Autodesk Inventor part; units mm, degrees
ref_plane "Work Plane1" through (0, 0, 0) normal (0.7071, 0.7071, 0) x (0, 0, 1)
ref_plane "XZ Plane" through (0, 0, 0) normal (0, 1, 0) x (-1, 0, 0)
ref_plane "XY Plane" through (0, 0, 0) normal (0, 0, 1) x (1, 0, 0)
sketch "Sketch1" plane through (0, 0, 0) normal (0, 0, 1) x (1, 0, 0)
  circle A0 centre (0, 0) radius 17.5
  dimension "d0" = 35
extrude "Extrusion1" add sketch "Sketch1" along normal blind 4
sketch "Sketch2" plane through (0, 0, 4) normal (0, 0, 1) x (1, 0, 0)
  circle A0 centre (0, 0) radius 7.625
  dimension "d3" = 15.25
extrude "Extrusion2" add sketch "Sketch2" along normal blind 5
chamfer "Chamfer1" distance 0.5 angle 45 1 edges at (-7.625, 0, 9)
sketch "Sketch3" plane through (0, 0, 0) normal (0, 0, -1) x (-1, 0, 0)
  line L0 (-7.4, -7.4) -> (7.4, -7.4)
  line L1 (7.4, -7.4) -> (7.4, 7.4)
  line L2 (7.4, 7.4) -> (-7.4, 7.4)
  line L3 (-7.4, 7.4) -> (-7.4, -7.4)
  line L4 (-7.4, -7.4) -> (7.4, 7.4) construction
  line L5 (7.4, -7.4) -> (-7.4, 7.4) construction
  point P0 (0, 0)
  dimension "d15" = 1.5
  dimension "d9" = 14.8
extrude "Extrusion3" cut sketch "Sketch3" against normal blind 1.2
sketch "Sketch4" plane through (0, 0, 0) normal (0, 0, -1) x (-1, 0, 0)
  line L0 (-7.4, -7.4) -> (-7.4, 7.4)
  circle A0 centre (-7.4, 7.4) radius 3
  point P0 (0, 0)
  dimension "d12" = 6
extrude "Extrusion4" cut sketch "Sketch4" against normal blind 3
sketch "Sketch5" plane through (0, 0, 0) normal (0, 0, -1) x (-1, 0, 0)
  circle A0 centre (-7.4, 7.4) radius 3
  line L0 (-7.4, 7.4) -> (-12.3744, 12.3744) construction
  circle A1 centre (0, 0) radius 17.5
  line L1 (-6.3393, 8.4607) -> (-11.3137, 13.435)
  line L2 (-13.435, 11.3137) -> (-8.4607, 6.3393)
  arc A2 (-8.4607, 6.3393) -> (-6.3393, 8.4607) centre (-7.4, 7.4) ccw
  arc A3 (-11.3137, 13.435) -> (-13.435, 11.3137) centre (-12.3744, 12.3744) ccw
  line L3 (0, -24.5) -> (0, 24.5)
  point P0 (-9.8872, 9.8872)
  point P1 (-13.3895, 11.2682)
  point P2 (-10.2978, 8.1765)
  point P3 (-8.1765, 10.2978)
  point P4 (-11.2682, 13.3895)
  dimension "d15" = 1.5
  dimension "d16" = 45
extrude "Extrusion5" cut sketch "Sketch5" against normal up to surface (3 mm away) contours A0 L2 A1 L1
pattern_circular "Circular Pattern1" count 4 over 360 about axis through (0, 0, -10) along (0, 0, 1) of "Extrusion4", "Extrusion5"
sketch "Sketch6" plane through (0, 0, 1.2) normal (0, 0, -1) x (-1, 0, 0)
  circle A0 centre (0, 0) radius 2.25
  dimension "d22" = 4.5
extrude "Extrusion6" cut sketch "Sketch6" against normal through all
ref_plane "Work Plane1" through (0, 0, 0) normal (0.7071, 0.7071, 0) x (0, 0, 1)
sketch "Sketch7" plane through (0, 0, 1.2) normal (0, 0, -1) x (-1, 0, 0)
  line L0 (7.4, 5.1639) -> (5.4, 5.1639)
  line L1 (5.4, 5.1639) -> (5.4, -5.1639)
  line L2 (5.4, -5.1639) -> (7.4, -5.1639)
  line L3 (7.4, -5.1639) -> (7.4, 5.1639)
  line L4 (7.4, 4.4) -> (7.4, -4.4)
  arc A0 (4.4, 7.4) -> (7.4, 4.4) centre (7.4, 7.4) ccw
  arc A1 (7.4, -4.4) -> (4.4, -7.4) centre (7.4, -7.4) ccw
  point P0 (0, 0)
  dimension "d26" = 2
extrude "Extrusion7" cut sketch "Sketch7" against normal up to surface (1.8 mm away)
pattern_circular "Circular Pattern2" count 4 over 360 about axis through (0, 0, -10) along (0, 0, 1) of "Extrusion7"
properties part number "chuck_v03_1.5inset" material "Polytetrafluoroethylene"
Source: CAD feature listing. Evaluate the final solid. Frame: model axes, mm. A direction names the side the tool comes from. Give positions to 0.01 mm unless a question says otherwise; leave off trailing zeros. Write each loop counter-clockwise with the first axis right and the second up, starting at its lowest first coordinate (ties: lowest second). Pieces come first, ordered by that corner, then holes.
1. Material intervals for line 1 along Y through (x, z) = (0, 7) (3 decimals); line 2 along X through (y, z) = (-3, 1.75); line 3 along Z through (x, y) = (-8, -4.5), sorted ascending.
2. First-contact query: pin 1 (5 mm diameter, centred on x = 2, z = 6, fed in from +Y); pin 2 (5.5 mm diameter, centred on x = -1.5, y = 0.5, fed in from -Z); pin 3 (6 mm diameter, centred on x = 0, y = -11.5, fed in from +Z). Flat tips, straight axial feed; report the tip coordinate or a pass-through.
3. Section query D-D (z = 4.75). Return the cut outline in (x, y) (3 decimals), then the cut area to 3 significant figures.
4. Section query A-A (y = 0). Return the cut outline in (x, z) (3 decimals), then the cut area to 3 significant figures.
5. Pull-direction query (Y, two-part tool) for faces 3 (the face through (0, 13, 0)), 4 (the face through (-6.05, 4.64, 6.22)), 5 (the face through (0, -5.4, 2)); classes: +Y half, -Y half, draft (parallel to the pull), parting line (faces both ways), or undercut.
6. Access query for faces 1 (the face through (12, 0, 0)), 2 (the face through (-11.865, -9.744, 1.479)). Directions: +Z, -Z, +X, -X, +Y, -Y. A direction counts if a zero-diameter tool reaches every point of the face in a straight line with its end or side. Return the directions, or none.
7. Section query C-C (z = 2.25). Count the separate pieces of the cut face and the enclosed holes in it, then the cut area to 3 significant figures.
Output values:
1. line 1: y = -7.625 to -2.25, 2.25 to 7.625
1. line 2: x = -17.24 to -7.4, -5.4 to 5.4, 7.4 to 17.24
1. line 3: z = 3 to 4
2. pin 1: stops at y = 17.49
2. pin 2: stops at z = 1.2
2. pin 3: stops at z = 4
3. outline: circle Ø15.25 at (0, 0); hole circle Ø4.5 at (0, 0)
3. area: 167 mm2
4. outline: (-17.5, 0) - (-7.4, 0) - (-7.4, 3) - (-5.4, 3) - (-5.4, 1.2) - (-2.25, 1.2) - (-2.25, 9) - (-7.125, 9) - (-7.625, 8.5) - (-7.625, 4) - (-17.5, 4) - close; (2.25, 1.2) - (5.4, 1.2) - (5.4, 3) - (7.4, 3) - (7.4, 0) - (17.5, 0) - (17.5, 4) - (7.625, 4) - (7.625, 8.5) - (7.125, 9) - (2.25, 9) - close
4. area: 156 mm2
5. face 3: draft
5. face 4: parting line
5. face 5: undercut
6. face 1: -Z, +X, -X, +Y, -Y
6. face 2: -Z
7. separate pieces: 5
7. enclosed holes: 1
7. area: 709 mm2
